The listing builds one solid part. Answer for the finished solid, in the listing's coordinates (mm). A direction names the side the tool comes from. Give positions to 0.01 mm unless a question says otherwise; leave off trailing zeros. Write each loop counter-clockwise with the first axis right and the second up, starting at its lowest first coordinate (ties: lowest second). Pieces come first, ordered by that corner, then holes. Notation, with made-up numbers: (6.25, 35.25) - (47.25, 35.25) arc R15 cw to (47.25, 63.25) - close; hole circle Ø8 at (48.5, 68.5). An arc over 180 degrees is marked (long way). Write each question's results on one line, items separated by ' | '. Start each with the question number.
Q1. Find the intervals of material crossed by probe 1 along X at (y, z) = (-8, 9) (3 decimals); probe 2 along X at (y, z) = (5.7, 0) (3 decimals); probe 3 along Y at (x, z) = (-6, 0), in increasing order.
Q2. For a pull along Y with two mould halves and no side action, classify faces 1 (the face through (15, 10, 0.049)), 2 (the face through (15.875, 9.5, 0.4)), 3 (the face through (14.909, 18.597, -4.13)) as pulls with the +Y half, pulls with the -Y half, needs draft (parallel to the pull), parting line crosses it, or undercut.
Q3. For faces 4 (the face through (15.25, 9.96, 0.67)), 5 (the face through (-0.196, 7.873, -1.748)), 6 (the face through (-0.07, 5.45, 1.5)), determine the directions among +Z, -Z, +X, -X, +Y, -Y from which every point of the face is accessible in a straight line to the end or side of a thin tool.
Q4. Flat-ended cylindrical pins translate along their axes: pin 1 Ø5 at (x, z) = (0, 0) entering from -Y; pin 2 Ø1 at (x, z) = (-7, -6.5) entering from -Y; pin 3 Ø2 at (x, y) = (-7, 8) entering from +Z; pin 4 Ø6 at (y, z) = (0, 0) entering from -X. Find the tip coordinate at first contact, or state that the pin passes through.
Q5. Section D-D (x = -8) is taken. Determine the outline of the cut face in (y, z), plus the area to 3 significant figures.
Q6. Section B-B (z = -9) is taken. Determine the outline of the cut face in (x, y) (3 decimals).
Q7. Section C-C (y = 7) is taken. Determine the outline of the cut face in (x, z) (3 decimals).
```python
from build123d import *

# Parameters (mm, degrees)
SKETCH1_W          = 13.97
SKETCH1_H          = 4.8006
SKETCH2_R          = 1.5
CUT_EXTRUDE1_DEPTH = 32.270123521
CUT_EXTRUDE2_DEPTH = 1.27


with BuildPart() as part:
    # Sketch1 → Revolve1 (revolve)
    with BuildSketch(Plane.XY, mode=Mode.PRIVATE) as revolve1_sk:
        with Locations((6.985, 5.6642)):
            Rectangle(SKETCH1_W, SKETCH1_H)
        Polygon((13.97, 8.0645), (13.97, 3.2639), (15.875, 3.2639), (15.875, 19.05), (13.97, 19.05), align=None)
        with Locations((-6.985, 5.6642)):
            Rectangle(SKETCH1_W, SKETCH1_H)
        Polygon((-15.875, 3.2639), (-13.97, 3.2639), (-13.97, 8.0645), (-13.97, 19.05), (-15.875, 19.05), align=None)
    revolve(revolve1_sk.sketch.rotate(Axis((-15.275524476, 0, 0), (1, 0, 0)), 90), axis=Axis((-15.275524476, 0, 0), (1, 0, 0)))

    # Sketch2 → Cut-Extrude1 (cut, through all)
    with BuildSketch(Plane(origin=(0, 0, 0), x_dir=(1, 0, 0), z_dir=(0, 1, 0))):
        with Locations(Location((0, 0, 0), (0, 0, 90))):
            Circle(SKETCH2_R)
    extrude(amount=CUT_EXTRUDE1_DEPTH, mode=Mode.SUBTRACT)

    # Sketch3 → Cut-Extrude2 (cut)
    with BuildSketch(Plane(origin=(15.875, 0, 0), x_dir=(0, 0, -1), z_dir=(1, 0, 0))):
        Polygon((0.253501878, 11.957106949), (0.330672017, 11.957106949), (0.330672017, 9.026337718), (0.819133555, 9.026337718), (0.819133555, 8.592149684), (0.330672017, 8.592149684), (0.330672017, 7.615226607), (-0.049242513, 7.615226607), (-0.049242513, 8.592149684), (-2.057362172, 8.592149684), align=None)
        Polygon((-0.049242513, 9.026337718), (-0.049242513, 10.863156629), (-1.310253464, 9.026337718), align=None, mode=Mode.SUBTRACT)
    extrude(amount=-CUT_EXTRUDE2_DEPTH, mode=Mode.SUBTRACT)


solid = part.part
```
Answers below:
1) probe 1: x = -15.875 to -13.97, 13.97 to 15.875 | probe 2: x = -15.875 to -1.5, 1.5 to 15.875 | probe 3: y = -8.06 to -3.26, 3.26 to 8.06
2) face 1: undercut | face 2: needs draft | face 3: parting line crosses it
3) face 4: +X | face 5: none | face 6: +Y
4) pin 1: stops at y = -8.06 | pin 2: stops at y = -5.39 | pin 3: stops at z = 4 | pin 4: passes through
5) outline: circle Ø16.13 at (0, 0); hole circle Ø6.53 at (0, 0) | area: 171 mm2
6) outline: (-15.875, -16.79) - (-13.97, -16.79) - (-13.97, 16.79) - (-15.875, 16.79) - close; (13.97, -16.79) - (15.875, -16.79) - (15.875, 16.79) - (13.97, 16.79) - close
7) outline: (-15.875, -17.717) - (-13.97, -17.717) - (-13.97, -4.005) - (13.97, -4.005) - (13.97, -17.717) - (15.875, -17.717) - (15.875, 17.717) - (13.97, 17.717) - (13.97, 4.005) - (-13.97, 4.005) - (-13.97, 17.717) - (-15.875, 17.717) - close; hole circle Ø3 at (0, 0)
